Input: dimensioned drawing with shaded views. Units: mm. Origin: part minimum x, y, z. A direction names the side the tool comes from. Give positions to 0.01 mm unless a question says otherwise; leave off trailing zeros. Order: outer loops, then holes, each group sorted by start corner. A loop starts at its lowest first (then second) coordinate and runs counter-clockwise, first axis right, second up. Notation, with made-up numbers: (21, 29.5) -> (58, 29.5) arc R23 ccw to (58, 43.5) -> close; hole circle Ø6 at (-2, -8). An arc over 180 degrees is marked (long way). Use CSV: the item, a comma, the result in double quotes.
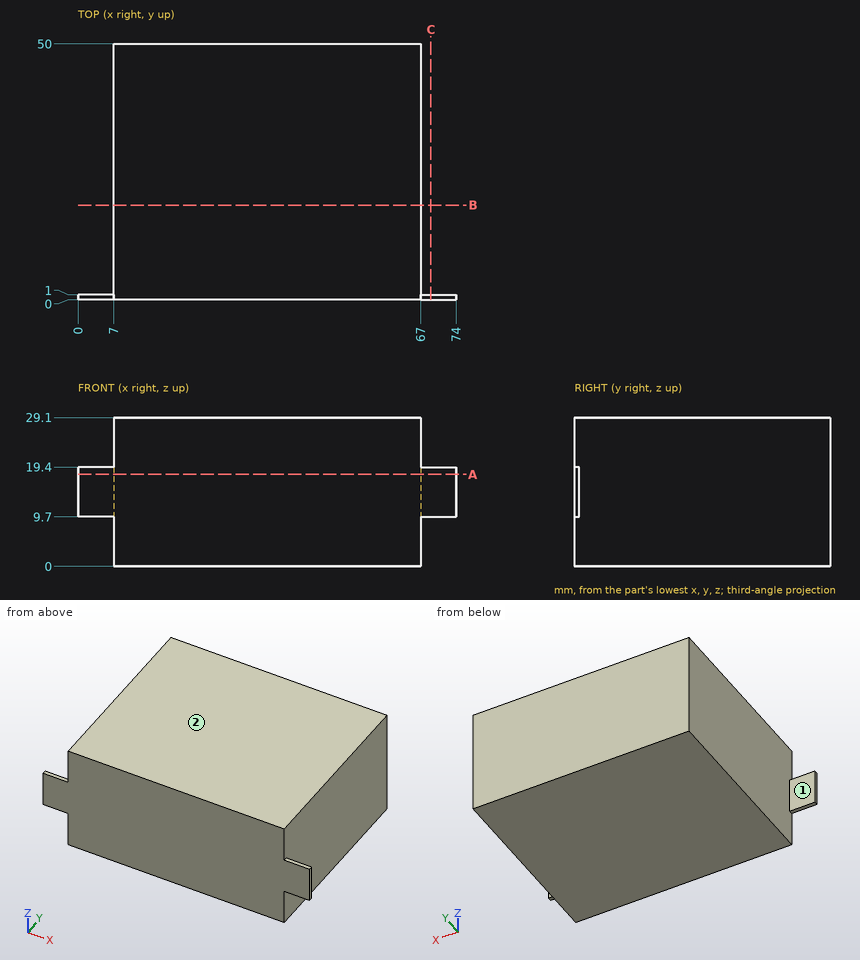
1. Section query A-A on z = 18. Return loops of the section in (x, y).
Answer below:
outline,"(0, 0) -> (74, 0) -> (74, 1) -> (67, 1) -> (67, 50) -> (7, 50) -> (7, 1) -> (0, 1) -> close"
2. Ray query, line 1 along Y through (x, z) = (5.5, 12.75); line 2 along X through (y, z) = (9.5, 16.5). Return the intervals inside material, ascending.
Answer below:
line 1,"y = 0 to 1"
line 2,"x = 7 to 67"
3. Access query for the marked faces 1 and 2. Directions: +Z, -Z, +X, -X, +Y, -Y. A direction counts if a zero-diameter tool reaches every point of the face in a straight line with its end or side. Return the directions, or none.
Answer below:
face 1,"+Z, -Z, -X, +Y"
face 2,"+Z, +X, -X, +Y, -Y"
4. Pin query (flat end, axial travel): P1, Ø0.5, axis at x = 70.5, y = 0.5, coming from the +Z side; P2, Ø1.5, axis at y = 43.5, z = 13, coming from the -X side; P3, Ø0.8, axis at x = 2.5, y = 0.5, coming from the -Z side. Return the tip coordinate at first contact, or that it passes through.
Answer below:
P1,"stops at z = 19.4"
P2,"stops at x = 7"
P3,"stops at z = 9.7"
5. Section query B-B on y = 18.5. Return loops of the section in (x, z).
Answer below:
outline,"(7, 0) -> (67, 0) -> (67, 29.1) -> (7, 29.1) -> close"
6. Section query C-C on x = 69. Return loops of the section in (y, z), plus the area to 3 significant figures.
Answer below:
outline,"(0, 9.7) -> (1, 9.7) -> (1, 19.4) -> (0, 19.4) -> close"
area,"9.70 mm²"
